from build123d import *

# Parameters (mm, degrees)
GENERAL_SHAPE_DEPTH             = 2
RETAINING_WALLS_DEPTH           = 14.5
EXTERIOR_MOUNTING_EDGE_DEPTH    = 2
REAR_WALL_DEPTH                 = 14.5
CUT_EXTRUDE2_DEPTH              = 51.801082666
CUT_EXTRUDE2_DEPTH_BACK         = 51.801082666
SKETCH35_R                      = 2.75
CIRPATTERN2_COUNT               = 4
EXTERIOR_MOUNTING_HOLE_D        = 2.4
SHOULDER_SCREW_MOUNTING_HOLES_D = 3.1
CUT_EXTRUDE1_REACH              = 50.195


with BuildPart() as part:
    # Sketch3 → General shape (new body)
    with BuildSketch(Plane(origin=(0, 0, 0), x_dir=(1, 0, 0), z_dir=(0, 1, 0))):
        Polygon((-32.5, -12.701010127), (-12.701010127, -32.5), (0, -19.798989873), (0, 0), (-19.798989873, 0), align=None)
    extrude(amount=GENERAL_SHAPE_DEPTH)

    # Sketch4 → Retaining walls (add)
    with BuildSketch(Plane(origin=(0, 2, 0), x_dir=(1, 0, 0), z_dir=(0, 1, 0))):
        Polygon((-19.798989873, 0), (-32.5, -12.701010127), (-31.085786438, -14.115223689), (-16.970562748, 0), align=None)
        Polygon((-14.115223689, -31.085786438), (0, -16.970562748), (0, -19.798989873), (-12.701010127, -32.5), align=None)
    extrude(amount=RETAINING_WALLS_DEPTH)

    # Sketch14 → Exterior mounting edge (add)
    with BuildSketch(Plane.XZ):
        Polygon((-19.798989873, 0), (-32.5, 12.701010127), (-32.5, 0), align=None)
        Polygon((0, 19.798989873), (0, 32.5), (-12.701010127, 32.5), align=None)
    extrude(amount=-EXTERIOR_MOUNTING_EDGE_DEPTH)

    # Sketch18 → Rear wall (add)
    with BuildSketch(Plane(origin=(0, 2, 0), x_dir=(1, 0, 0), z_dir=(0, 1, 0))):
        Polygon((-16.970562748, 0), (0, -16.970562748), (-1.414213562, -18.384776311), (-18.384776311, -1.414213562), align=None)
    extrude(amount=REAR_WALL_DEPTH)

    # Sketch35 → Cut-Extrude2 (cut, two sides: drawn at the far end of the back side and taken through both)
    with BuildSketch(Plane(origin=(-9.899494937, 0, -9.899494937), x_dir=(-0.7071067811865475, 0, 0.7071067811865477), z_dir=(-0.7071067811865477, 0, -0.7071067811865475)).offset(-CUT_EXTRUDE2_DEPTH_BACK)):
        with Locations((25.5, 9.25)):
            Circle(SKETCH35_R)
    extrude(amount=CUT_EXTRUDE2_DEPTH + CUT_EXTRUDE2_DEPTH_BACK, mode=Mode.SUBTRACT)


with BuildPart() as cirpattern2_1:
    # CirPattern2: pattern copy
    add(part.part.rotate(Axis((0, 0, 0), (0, 1, 0)), 1 * 360 / CIRPATTERN2_COUNT))


with BuildPart() as cirpattern2_2:
    # CirPattern2: pattern copy
    add(part.part.rotate(Axis((0, 0, 0), (0, 1, 0)), 2 * 360 / CIRPATTERN2_COUNT))


with BuildPart() as cirpattern2_3:
    # CirPattern2: pattern copy
    add(part.part.rotate(Axis((0, 0, 0), (0, 1, 0)), 3 * 360 / CIRPATTERN2_COUNT))

    # Combine1: union CirPattern2_1, CirPattern2_2, part
    add(cirpattern2_1.part)
    add(cirpattern2_2.part)
    add(part.part)

    # Exterior mounting hole (through all)
    with Locations(Plane(origin=(0, 2, 0), x_dir=(1, 0, 0), z_dir=(0, 1, 0))):
        with Locations((-25.1, 0), (25.1, 0)):
            Hole(EXTERIOR_MOUNTING_HOLE_D / 2)

    # Shoulder screw mounting holes (through all)
    with Locations(Plane(origin=(0, 2, 0), x_dir=(1, 0, 0), z_dir=(0, 1, 0))):
        with Locations((0, -25.1), (0, 25.1)):
            Hole(SHOULDER_SCREW_MOUNTING_HOLES_D / 2)

    # Sketch23 → Cut-Extrude1 (cut, up to next)
    with BuildSketch(Plane(origin=(0, 2, 0), x_dir=(1, 0, 0), z_dir=(0, 1, 0)), mode=Mode.PRIVATE) as cut_extrude1_sk1:
        Polygon((0, 16.970562748), (-16.970562748, 0), (0, -16.970562748), (16.970562748, 0), align=None)
    cut_extrude1_tool1 = extrude(cut_extrude1_sk1.sketch, amount=-CUT_EXTRUDE1_REACH, mode=Mode.PRIVATE) & cirpattern2_3.part
    # Sketch23 → Cut-Extrude1 (cut, up to next)
    with BuildSketch(Plane(origin=(0, 2, 0), x_dir=(1, 0, 0), z_dir=(0, 1, 0)), mode=Mode.PRIVATE) as cut_extrude1_sk2:
        Polygon((31.085786438, 14.115223689), (18.384776311, 1.414213562), (1.414213562, 18.384776311), (14.115223689, 31.085786438), align=None)
    cut_extrude1_tool2 = extrude(cut_extrude1_sk2.sketch, amount=-CUT_EXTRUDE1_REACH, mode=Mode.PRIVATE) & cirpattern2_3.part
    # Sketch23 → Cut-Extrude1 (cut, up to next)
    with BuildSketch(Plane(origin=(0, 2, 0), x_dir=(1, 0, 0), z_dir=(0, 1, 0)), mode=Mode.PRIVATE) as cut_extrude1_sk3:
        Polygon((-18.384776311, 1.414213562), (-31.085786438, 14.115223689), (-14.115223689, 31.085786438), (-1.414213562, 18.384776311), align=None)
    cut_extrude1_tool3 = extrude(cut_extrude1_sk3.sketch, amount=-CUT_EXTRUDE1_REACH, mode=Mode.PRIVATE) & cirpattern2_3.part
    # Sketch23 → Cut-Extrude1 (cut, up to next)
    with BuildSketch(Plane(origin=(0, 2, 0), x_dir=(1, 0, 0), z_dir=(0, 1, 0)), mode=Mode.PRIVATE) as cut_extrude1_sk4:
        Polygon((-1.414213562, -18.384776311), (-14.115223689, -31.085786438), (-31.085786438, -14.115223689), (-18.384776311, -1.414213562), align=None)
    cut_extrude1_tool4 = extrude(cut_extrude1_sk4.sketch, amount=-CUT_EXTRUDE1_REACH, mode=Mode.PRIVATE) & cirpattern2_3.part
    # Sketch23 → Cut-Extrude1 (cut, up to next)
    with BuildSketch(Plane(origin=(0, 2, 0), x_dir=(1, 0, 0), z_dir=(0, 1, 0)), mode=Mode.PRIVATE) as cut_extrude1_sk5:
        Polygon((14.115223689, -31.085786438), (1.414213562, -18.384776311), (18.384776311, -1.414213562), (31.085786438, -14.115223689), align=None)
    cut_extrude1_tool5 = extrude(cut_extrude1_sk5.sketch, amount=-CUT_EXTRUDE1_REACH, mode=Mode.PRIVATE) & cirpattern2_3.part
    add(cut_extrude1_tool1.solids().sort_by_distance((0, 2, 0))[0], mode=Mode.SUBTRACT)
    add(cut_extrude1_tool2.solids().sort_by_distance((16.25, 2, -16.25))[0], mode=Mode.SUBTRACT)
    add(cut_extrude1_tool3.solids().sort_by_distance((-16.25, 2, -16.25))[0], mode=Mode.SUBTRACT)
    add(cut_extrude1_tool4.solids().sort_by_distance((-16.25, 2, 16.25))[0], mode=Mode.SUBTRACT)
    add(cut_extrude1_tool5.solids().sort_by_distance((16.25, 2, 16.25))[0], mode=Mode.SUBTRACT)


solid = cirpattern2_3.part
Can you work these out from the model? Positions are in its coordinate system, mm. A direction names the side the tool comes from. Give positions to 0.01 mm unless a question says otherwise; leave off trailing zeros. Loops run counter-clockwise (first coordinate to the right, second up) from the corner with the lowest first, then second, coordinate; pieces in that order, holes last. Notation, with made-up numbers: M 44.5,-9.5 L 82.5,-9.5 A33 cw 82.5,23.5 Z; hole C 68.5,40.25 d6. An arc over 180 degrees is marked long. One line per item, written item: value. Start each with the question number.
1) If we section it at A-A, the plane y = 1: Give the number of separate pieces and of enclosed holes in the cut face, and give its area (3 significant figures).
2) If I drill on line 1 (Z direction, x = 0, y = 1); line 2 (X direction, y = 9.5, z = 11.5); line 3 (Z direction, x = 6.5, y = 14), over which ranges is the centre line in solid material (lowest first)? Write a range as [from, to].
3) On a 3-axis mill with a long thin cutter (end or side, diameter ignored), from which of +Z, -Z, +X, -X, +Y, -Y can I reach the whole of each face in a straight line? I mean faces 4 (the face through (7.4, 16.5, -9.8)), 5 (the face through (8.6, 8.13, -8.37)). Say none if no direction works.
4) I'm going to push flat-ended pins straight in: pin 1 (1.9 mm diameter, centred on x = -25.1, z = 0, fed in from +Y); pin 2 (5 mm diameter, centred on x = 0, z = -25.1, fed in from +Y); pin 3 (5 mm diameter, centred on y = 12.5, z = 25, fed in from -X); pin 4 (8 mm diameter, centred on x = 18, y = 3.5, fed in from +Z). Where does each tip first touch, or does it pass through?
5) Thinking about a two-plate mould opening in Z: for faces 1 (the face through (-28.28, 11.57, -9.87)), 2 (the face through (31.8, 8.1, -13.4)), 3 (the face through (0, 2, 29)), which applies, +Z half, -Z half, draft (parallel to the pull), parting line (faces both ways), or undercut?
6) If we section it at C-C, the plane x = -3: Write out the boundary of the cut face in (y, z), and give its area (3 significant figures).
Completed:
1. separate pieces: 1
1. enclosed holes: 5
1. area: 1,120 mm^2
2. line 1: z = [-32.5, -26.65], [-23.55, -16.97], [16.97, 23.55], [26.65, 32.5]
2. line 2: x = [-31.3, -28.47], [-8.3, -5.47], [5.47, 8.3], [28.47, 31.3]
2. line 3: z = [-26.3, -23.47], [-13.3, -10.47], [10.47, 13.3], [23.47, 26.3]
3. face 4: +Z, -Z, +X, -X, +Y
3. face 5: +Y, -Y
4. pin 1: passes through
4. pin 2: stops at y = 2
4. pin 3: stops at x = -10.53
4. pin 4: stops at z = 31.2
5. face 1: undercut
5. face 2: -Z half
5. face 3: draft
6. outline: M 0,-32.5 L 2,-32.5 L 2,-22.8 L 16.5,-22.8 L 16.5,-19.97 L 0,-19.97 Z; M 0,-16.8 L 16.5,-16.8 L 16.5,-13.97 L 0,-13.97 Z; M 0,13.97 L 16.5,13.97 L 16.5,16.8 L 0,16.8 Z; M 0,19.97 L 16.5,19.97 L 16.5,22.8 L 2,22.8 L 2,32.5 L 0,32.5 Z
6. area: 225 mm^2
